For this review, take the finished solid that the model builds, in its own axes (mm). A direction names the side the tool comes from. Round coordinates to 2 decimals unless told otherwise and drop trailing zeros. Loops run counter-clockwise (first coordinate to the right, second up) from the corner with the lowest first, then second, coordinate; pieces in that order, holes last.
```python
from build123d import *

# Parameters (mm, degrees)
BOSS_EXTRUDE1_START            = 6.35
BOSS_EXTRUDE1_OUTLINE_W        = 200
BOSS_EXTRUDE1_OUTLINE_H        = 6.35
BOSS_EXTRUDE1_DEPTH            = 37.301670771
BOSS_EXTRUDE1_2_OUTLINE_W      = 10
BOSS_EXTRUDE1_2_OUTLINE_H      = 6.35
BOSS_EXTRUDE1_2_DEPTH          = 50.001670771
BOSS_EXTRUDE1_START_2          = 20.000835386
BOSS_EXTRUDE1_3_OUTLINE_W      = 6.35
BOSS_EXTRUDE1_3_OUTLINE_H      = 6.35
BOSS_EXTRUDE1_3_DEPTH          = 10
F_1_16_0_0625_DIAMETER_HOLE1_D = 1.5875


# Read off the part's stored shape, not the designer's step: Boss-Extrude1
with BuildPart() as part:
    # Boss-Extrude1 outline → Boss-Extrude1 (new body)
    with BuildSketch(Plane(origin=(0, 0, 0), x_dir=(1, 0, 0), z_dir=(0, 1, 0)).offset(BOSS_EXTRUDE1_START)):
        with Locations((100, -3.175)):
            Rectangle(BOSS_EXTRUDE1_OUTLINE_W, BOSS_EXTRUDE1_OUTLINE_H)
    extrude(amount=BOSS_EXTRUDE1_DEPTH)

    # Boss-Extrude1 2 outline → Boss-Extrude1 2 (add)
    with BuildSketch(Plane(origin=(0, 0, 0), x_dir=(1, 0, 0), z_dir=(0, 1, 0))):
        with Locations((25, -3.175)):
            Rectangle(BOSS_EXTRUDE1_2_OUTLINE_W, BOSS_EXTRUDE1_2_OUTLINE_H)
        with Locations((45, -3.175)):
            Rectangle(BOSS_EXTRUDE1_2_OUTLINE_W, BOSS_EXTRUDE1_2_OUTLINE_H)
        with Locations((5, -3.175)):
            Rectangle(BOSS_EXTRUDE1_2_OUTLINE_W, BOSS_EXTRUDE1_2_OUTLINE_H)
        with Locations((65, -3.175)):
            Rectangle(BOSS_EXTRUDE1_2_OUTLINE_W, BOSS_EXTRUDE1_2_OUTLINE_H)
        with Locations((85, -3.175)):
            Rectangle(BOSS_EXTRUDE1_2_OUTLINE_W, BOSS_EXTRUDE1_2_OUTLINE_H)
        with Locations((105, -3.175)):
            Rectangle(BOSS_EXTRUDE1_2_OUTLINE_W, BOSS_EXTRUDE1_2_OUTLINE_H)
        with Locations((125, -3.175)):
            Rectangle(BOSS_EXTRUDE1_2_OUTLINE_W, BOSS_EXTRUDE1_2_OUTLINE_H)
        with Locations((145, -3.175)):
            Rectangle(BOSS_EXTRUDE1_2_OUTLINE_W, BOSS_EXTRUDE1_2_OUTLINE_H)
        with Locations((165, -3.175)):
            Rectangle(BOSS_EXTRUDE1_2_OUTLINE_W, BOSS_EXTRUDE1_2_OUTLINE_H)
        with Locations((185, -3.175)):
            Rectangle(BOSS_EXTRUDE1_2_OUTLINE_W, BOSS_EXTRUDE1_2_OUTLINE_H)
    extrude(amount=BOSS_EXTRUDE1_2_DEPTH)

    # Boss-Extrude1 3 outline → Boss-Extrude1 3 (add)
    with BuildSketch(Plane(origin=(0, 0, 0), x_dir=(1, 0, 0), z_dir=(0, 1, 0)).offset(BOSS_EXTRUDE1_START_2)):
        with Locations((-3.175, -3.175)):
            Rectangle(BOSS_EXTRUDE1_3_OUTLINE_W, BOSS_EXTRUDE1_3_OUTLINE_H)
        with Locations((203.175, -3.175)):
            Rectangle(BOSS_EXTRUDE1_3_OUTLINE_W, BOSS_EXTRUDE1_3_OUTLINE_H)
    extrude(amount=BOSS_EXTRUDE1_3_DEPTH)

    # 1/16 (0.0625) Diameter Hole1 (through all)
    with Locations(Plane.XY.offset(6.35)):
        with Locations((10, 43.651670771), (20, 43.651670771), (20, 6.35), (10, 6.35), (29.999999878, 43.651670771), (39.999999878, 43.651670771), (39.999999878, 6.35), (29.999999878, 6.35), (49.999999756, 43.651670771), (59.999999756, 43.651670771), (59.999999756, 6.35), (49.999999756, 6.35), (69.999999634, 43.651670771), (79.999999634, 43.651670771), (79.999999634, 6.35), (69.999999634, 6.35), (89.999999512, 43.651670771), (99.999999512, 43.651670771), (99.999999512, 6.35), (89.999999512, 6.35), (109.99999939, 43.651670771), (119.99999939, 43.651670771), (119.99999939, 6.35), (109.99999939, 6.35), (129.999999268, 43.651670771), (139.999999268, 43.651670771), (139.999999268, 6.35), (129.999999268, 6.35), (149.999999146, 43.651670771), (159.999999146, 43.651670771), (159.999999146, 6.35), (149.999999146, 6.35), (169.999999024, 43.651670771), (179.999999024, 43.651670771), (179.999999024, 6.35), (169.999999024, 6.35), (190, 43.651670771), (190, 6.35), (200, 20.000835386), (200, 30.000835386), (0, 30.000835386), (0, 20.000835386)):
            Hole(F_1_16_0_0625_DIAMETER_HOLE1_D / 2)


solid = part.part
```
(1) Add section A-A (x = 14). Give the boundary of the cut face in (y, z), plus the area to 3 significant figures.
(2) The part is to be moulded in two halves that separate along X. For faces 1 (the flat face through (206.35, 25, 3)), 2 (the flat face through (175, 6.35, 3)), 3 (the flat face through (25, 50.002, 3)), say which applies: pulls with the +X half, pulls with the -X half, needs draft (parallel to the pull), parting line crosses it, or undercut.
(3) For L1, parallel to X at y = 34.5, z = 3.75; L2, parallel to Y at x = 56, z = 3.5; L3, parallel to Y at x = 10.5, z = 1.25, list the stretches that pass through material, from the lowest coordinate up.
(4) For faces 4 (the flat face through (190, 47, 3)), 5 (the flat face through (10, 3, 3)), 6 (the flat face through (165, 0, 3)), 7 (the flat face through (90, 47, 3)), 8 (the flat face through (-4, 30.001, 3)), list the 3-axis set-ups (+Z, -Z, +X, -X, +Y, -Y) from which the entire face can be reached by the end or side of a thin tool; tool diameter is ignored.
(5) Add section B-B (y = 39). Give the boundary of the cut face in (x, z).
(6) Insertion check: pin 1 Ø1.7 at (y, z) = (1.5, 3.5) entering from -X; pin 2 Ø1.7 at (y, z) = (3.5, 3.5) entering from +X; pin 3 Ø1.8 at (x, y) = (180, 43.65) entering from +Z; pin 4 Ø3 at (x, z) = (116.5, 3.5) entering from -Y. Each pin has a flat end and moves straight along its axis. Give the tip position at first contact, or say it passes through.
Outcome:
1. outline: (6.35, 0) - (43.65, 0) - (43.65, 6.35) - (6.35, 6.35) - close
1. area: 237 mm2
2. face 1: pulls with the +X half
2. face 2: undercut
2. face 3: needs draft
3. L1: x = 0 to 200
3. L2: y = 6.35 to 43.65
3. L3: y = 6.97 to 43.04
4. face 4: +Z, -Z, +X, +Y
4. face 5: +Z, -Z, -Y
4. face 6: +Z, -Z, +X, -X, -Y
4. face 7: +Z, -Z, +Y
4. face 8: +Z, -Z, -X, +Y
5. outline: (0, 0) - (200, 0) - (200, 6.35) - (0, 6.35) - close
6. pin 1: stops at x = 0
6. pin 2: stops at x = 190
6. pin 3: stops at z = 6.35
6. pin 4: stops at y = 6.35
